Autodesk Inventor part; units mm, degrees
ref_plane "YZ Plane" through (0, 0, 0) normal (1, 0, 0) x (0, 1, 0)
ref_plane "XZ Plane" through (0, 0, 0) normal (0, 1, 0) x (-1, 0, 0)
ref_plane "XY Plane" through (0, 0, 0) normal (0, 0, 1) x (1, 0, 0)
sketch "Sketch1" plane through (0, 0, 0) normal (0, 0, 1) x (1, 0, 0)
  line L0 (85.6, 13.1) -> (-85.6, 13.1)
  line L1 (-85.6, 13.1) -> (-85.6, -13.1)
  line L2 (-85.6, -13.1) -> (85.6, -13.1)
  line L3 (85.6, -13.1) -> (85.6, 13.1)
  line L4 (85.6, 13.1) -> (-85.6, -13.1) construction
  line L5 (-85.6, 13.1) -> (85.6, -13.1) construction
  point P0 (0, 0)
  dimension "d0" = 171.2
  dimension "d1" = 26.2
extrude "Extrusion1" add sketch "Sketch1" along normal blind 11
sketch "Sketch2" plane through (85.6, -13.1, 0) normal (1, 0, 0) x (0, 0, -1)
  line L0 (0, 0) -> (0, 26.2)
  line L1 (0, 26.2) -> (-11, 26.2)
  line L2 (-11, 0) -> (-11, 26.2)
  line L3 (0, 0) -> (-11, 0)
  line L4 (-11, 26.2) -> (-11, 0)
  line L5 (-11, 26.2) -> (-5, 26.2)
  line L6 (-5, 26.2) -> (-5, 23.2)
  line L7 (-5, 23.2) -> (-11, 23.2)
  line L8 (-11, 23.2) -> (-11, 26.2)
  line L9 (-11, 23.2) -> (-8, 23.2)
  line L10 (-8, 23.2) -> (-8, 20.2)
  line L11 (-8, 20.2) -> (-11, 20.2)
  line L12 (-11, 20.2) -> (-11, 23.2)
  line L13 (-11, 26.2) -> (-5, 26.2)
  line L14 (-5, 26.2) -> (-5, 10.2)
  line L15 (-5, 10.2) -> (-11, 10.2)
  line L16 (-11, 10.2) -> (-11, 26.2)
  line L17 (-11, 10.2) -> (-5, 10.2)
  line L18 (-5, 10.2) -> (-5, 13.2)
  line L19 (-5, 13.2) -> (-11, 13.2)
  line L20 (-11, 13.2) -> (-11, 10.2)
  line L21 (-11, 13.2) -> (-8, 13.2)
  line L22 (-8, 13.2) -> (-8, 16.2)
  line L23 (-8, 16.2) -> (-11, 16.2)
  line L24 (-11, 16.2) -> (-11, 13.2)
  point P0 (0, 13.1)
  point P1 (-11, 20.2)
  dimension "d4" = 6
  dimension "d5" = 3
  dimension "d6" = 3
  dimension "d7" = 3
  dimension "d8" = 16
  dimension "d9" = 3
  dimension "d10" = 3
  dimension "d11" = 3
extrude "Extrusion2" cut sketch "Sketch2" against normal blind 168.2 contours L14 L19 L22 L23 L2 L11 L10 L7
fillet "Fillet1" radius 2 5 edges at (85.6, 10.1, 11) (85.6, -5, 11) (-85.6, 0, 11) (85.6, 0, 0) (-85.6, 0, 0)
sketch "Sketch4" plane through (-83.6, -13.1, 0) normal (0, -1, 0) x (1, 0, 0)
  arc A0 (-2, 2) -> (0, 0) centre (0, 2) ccw
  line L0 (0, 0) -> (167.2, 0)
  arc A1 (167.2, 0) -> (169.2, 2) centre (167.2, 2) ccw
  line L1 (169.2, 2) -> (169.2, 9)
  arc A2 (169.2, 9) -> (167.2, 11) centre (167.2, 9) ccw
  line L2 (0, 11) -> (167.2, 11)
  arc A3 (0, 11) -> (-2, 9) centre (0, 9) ccw
  line L3 (-2, 2) -> (-2, 9)
  circle A4 centre (159.2, 5.5) radius 4.1
  circle A5 centre (152.2, 5.5) radius 2.15
  line L4 (152.2, 7.65) -> (155.7089, 7.65)
  line L5 (152.2, 3.35) -> (155.7089, 3.35)
  circle A6 centre (15, 5.5) radius 4.1
  circle A7 centre (8, 5.5) radius 2.15
  line L6 (8, 3.35) -> (11.5089, 3.35)
  line L7 (8, 7.65) -> (11.5089, 7.65)
  point P0 (83.6, 0)
  point P1 (169.2, 5.5)
  point P2 (12.2407, 8.5325)
  point P3 (8.4381, 3.3951)
  point P4 (11.1965, 3.9692)
  point P5 (-2, 5.5)
  dimension "d19" = 8.2
  dimension "d20" = 4.3
  dimension "d21" = 7
  dimension "d22" = 0
  dimension "d23" = 10
  dimension "d24" = 8.2
  dimension "d25" = 4.3
  dimension "d26" = 7
  dimension "d27" = 10
  dimension "d28" = 0
  dimension "d40" = 0
extrude "Extrusion4" cut sketch "Sketch4" against normal blind 5.2 contours A4 | A4 L5 A5 L4 | A5 | A6 | A6 L6 A7 L7 | A7
sketch "Sketch5" plane through (-83.6, -13.1, 0) normal (0, -1, 0) x (1, 0, 0)
  arc A0 (8, 7.65) -> (8, 3.35) centre (8, 5.5) ccw
  arc A1 (11.5089, 3.35) -> (11.5089, 7.65) centre (15, 5.5) ccw
  arc A2 (152.2, 7.65) -> (152.2, 3.35) centre (152.2, 5.5) ccw
  line L0 (152.2, 7.65) -> (155.7089, 7.65)
  arc A3 (155.7089, 3.35) -> (155.7089, 7.65) centre (159.2, 5.5) ccw
  line L1 (155.7089, 3.35) -> (152.2, 3.35)
  arc A4 (-2, 2) -> (0, 0) centre (0, 2) ccw
  line L2 (0, 0) -> (167.2, 0)
  arc A5 (167.2, 0) -> (169.2, 2) centre (167.2, 2) ccw
  line L3 (169.2, 2) -> (169.2, 9)
  arc A6 (169.2, 9) -> (167.2, 11) centre (167.2, 9) ccw
  line L4 (0, 11) -> (167.2, 11)
  arc A7 (0, 11) -> (-2, 9) centre (0, 9) ccw
  line L5 (-2, 2) -> (-2, 9)
  circle A8 centre (8, 5.5) radius 4.1
  line L6 (8, 9.6) -> (15, 9.6)
  line L7 (8, 1.4) -> (15, 1.4)
  arc A9 (11.5089, 3.35) -> (11.5089, 7.65) centre (15, 5.5) ccw
  circle A10 centre (152.2, 5.5) radius 4.1
  line L8 (152.2, 9.6) -> (159.2, 9.6)
  line L9 (159.2, 1.4) -> (152.2, 1.4)
  line L10 (8, 7.65) -> (11.5089, 7.65)
  line L11 (11.5089, 3.35) -> (8, 3.35)
  arc A11 (8, 7.65) -> (8, 3.35) centre (8, 5.5) ccw
  point P0 (83.6, 0)
  point P1 (19.1, 5.5)
  point P2 (19.1, 5.5)
  point P3 (5.85, 5.5)
  point P4 (150.05, 5.5)
  point P5 (12.4867, 2.2607)
  point P6 (12.4867, 8.7393)
  point P7 (96.275, 2.2698)
  point P8 (96.275, 8.7302)
  point P9 (5.85, 5.5)
  point P10 (155.6911, 7.65)
  point P11 (155.6911, 3.35)
  point P12 (11.4911, 3.35)
  point P13 (11.4911, 7.65)
  dimension "d32" = 8.2
  dimension "d33" = 0
  dimension "d35" = 8.2
  dimension "d36" = 0
  dimension "d42" = 0
  dimension "d43" = 0
extrude "Extrusion5" cut sketch "Sketch5" along normal blind 3.2 from surface at -5.2 contours L10 A8 L11 A0 | A0 L11 A8 L10 | A8 L6 A1 L10 | L11 A1 L7 A8 | L0 A10 L1 A2 | A2 L1 A10 L0 | A10 L8 A3 L0 | L1 A3 L9 A10
properties part number "module-slot" material "PC/ABS Plastic"
The listing builds one solid part. Answer for the finished solid, in the listing's coordinates (mm). A direction names the side the tool comes from. Coordinates: 2 decimals unless noted, no trailing zeros. Order: outer loops, then holes, each group sorted by start corner. A loop starts at its lowest first (then second) coordinate and runs counter-clockwise, first axis right, second up. Notation, with made-up numbers: (73.25, 57) -> (95.25, 57) arc R24 ccw to (95.25, 67) -> close; hole circle Ø11 at (66, 45). An arc over 180 degrees is marked (long way). Answer in a Markdown table with one row per item. Add a question column.
Item 1: Which of the six approach directions +Z, -Z, +X, -X, +Y, -Y give full straight-line access (tool end or side, diameter ignored) to faces 1 (the face through (3, 7.1, 9)), 2 (the face through (1, 13.1, 5)), 3 (the face through (3, 10.1, 6)), 4 (the face through (-79.7, -9.5, 5.4)), 5 (the face through (-85.6, 0, 5))?
Item 2: Find the intervals of material crossed by L1, parallel to X at y = -9.45, z = 5.5; L2, parallel to Y at x = -6.5, z = 5.25; L3, parallel to Z at x = -1, y = 7.5, in increasing order. Write a range as from..to.
Item 3: Determine the mould class of faces 6 (the face through (3, 3.1, 9)), 7 (the face through (85.6, -0.2, 5.5)), 8 (the face through (-64.5, -11.1, 5.4)) for opening direction X: +X half, -X half, draft (parallel to the pull), parting line (faces both ways), or undercut.
Item 4: This flat-tipped pin is pushed along its axis until it touches: P1, Ø4, axis at y = 8, z = 6.5, coming from the +X side. Where does it stop, or does it pass through?
Item 5: Find section A-A (x = 31). Write down the section's boundary in (y, z), then the cut area to 3 significant figures.
Result set:
| question | item | result |
|---|---|---|
| 1 | face 1 | +Z, +X |
| 1 | face 2 | +Z, -Z, +X, -X, +Y |
| 1 | face 3 | +X |
| 1 | face 4 | none |
| 1 | face 5 | +Z, -Z, -X, +Y, -Y |
| 2 | L1 | x = -85.6..-79.7, -64.5..64.5, 79.7..85.6 |
| 2 | L2 | y = -13.1..0.1, 10.1..13.1 |
| 2 | L3 | z = 0..5, 8..11 |
| 3 | face 6 | draft |
| 3 | face 7 | +X half |
| 3 | face 8 | undercut |
| 4 | P1 | stops at x = 85.6 |
| 5 | outline | (-13.1, 0) -> (13.1, 0) -> (13.1, 11) -> (7.1, 11) -> (7.1, 8) -> (10.1, 8) -> (10.1, 5) -> (0.1, 5) -> (0.1, 8) -> (3.1, 8) -> (3.1, 11) -> (-13.1, 11) -> close |
| 5 | area | 246 mm² |
